Read the model definition and answer for the solid it produces. Units are mm, in the model's axes. A direction names the side the tool comes from. Coordinates: 2 decimals unless noted, no trailing zeros. Loops run counter-clockwise (first coordinate to the right, second up) from the corner with the lowest first, then second, coordinate; pieces in that order, holes last.
Q1. Section B-B (z = -7) is taken. Give the vertices of the cut face in (x, y).
Q2. The mould has two halves that part along Z. Classify faces 1 (the face through (-1, 0, -9)), 2 (the face through (13, -13, 0)), 3 (the face through (0, -13, 9.3)): pulls with the +Z half, pulls with the -Z half, needs draft (parallel to the pull), parting line crosses it, or undercut.
Q3. Which of the six approach directions +Z, -Z, +X, -X, +Y, -Y give full straight-line access (tool end or side, diameter ignored) to faces 4 (the face through (0, -13, -8.5)), 5 (the face through (-13.4, -11.4, -1.2)), 6 (the face through (-1, -26, -9))?
Q4. Straight lines are drawn through the part: line 1 (Z direction, x = -13.3, y = -13); line 2 (X direction, y = -19, z = 4); line 3 (Z direction, x = -3, y = -20.25). For each, find the intervals that lie inside material, in ascending order.
Q5. Section C-C (y = -19.5) is taken. Give the vertices of the cut face in (x, z).
Q6. Section D-D (z = 0) is taken. Give the vertices of the cut face in (x, y), then the cut area to 3 significant figures.
Q7. Section A-A (x = -2) is taken. Give the vertices of the cut face in (y, z).
from build123d import *

# Parameters (mm, degrees)
F0_W     = 27.6
F0_H     = 18.6
F0_W_2   = 26
F0_H_2   = 17
F1_DEPTH = 26
F2_R     = 2
F3_DEPTH = 3


with BuildPart() as f1:
    # F0 (on Front) → F1 (new body)
    with BuildSketch(Plane.XZ):
        Rectangle(F0_W, F0_H)
        Rectangle(F0_W_2, F0_H_2, mode=Mode.SUBTRACT)
    extrude(amount=F1_DEPTH)

    # F2 (on face) → F3 (cut)
    with BuildSketch(Plane(origin=(-13.8, 0, 0), x_dir=(0, -1, 0), z_dir=(-1, 0, 0))):
        with Locations((13, 0)):
            Circle(F2_R)
    extrude(amount=-F3_DEPTH, mode=Mode.SUBTRACT)


solid = f1.part
Numbers:
1. outline: (-13.8, -26) - (-13, -26) - (-13, 0) - (-13.8, 0) - close; (13, -26) - (13.8, -26) - (13.8, 0) - (13, 0) - close
2. face 1: needs draft
2. face 2: undercut
2. face 3: pulls with the +Z half
3. face 4: +Y, -Y
3. face 5: -X
3. face 6: +Z, -Z, +X, -X, -Y
4. line 1: z = -9.3 to -2, 2 to 9.3
4. line 2: x = -13.8 to -13, 13 to 13.8
4. line 3: z = -9.3 to -8.5, 8.5 to 9.3
5. outline: (-13.8, -9.3) - (13.8, -9.3) - (13.8, 9.3) - (-13.8, 9.3) - close; hole (-13, -8.5) - (13, -8.5) - (13, 8.5) - (-13, 8.5) - close
6. outline: (-13.8, -26) - (-13, -26) - (-13, -15) - (-13.8, -15) - close; (-13.8, -11) - (-13, -11) - (-13, 0) - (-13.8, 0) - close; (13, -26) - (13.8, -26) - (13.8, 0) - (13, 0) - close
6. area: 38.4 mm2
7. outline: (-26, -9.3) - (0, -9.3) - (0, -8.5) - (-26, -8.5) - close; (-26, 8.5) - (0, 8.5) - (0, 9.3) - (-26, 9.3) - close
